from build123d import *

# Parameters (mm, degrees)
BOX015_W                  = 10
BOX015_H                  = 10
BOX015_DEPTH              = 19
BOX014_W                  = 10
BOX014_H                  = 10
BOX014_DEPTH              = 19
CHAMFER023006003002_SIZE2 = 9
CHAMFER023006003002_SIZE  = 10
TUBE_R                    = 4
TUBE_R_2                  = 2
TUBE_DEPTH                = 10


with BuildPart() as cube015:
    # Box015 → Box015 (new body)
    with BuildSketch(Plane(origin=(-8.5, 12, 8.5), x_dir=(1, 0, 0), z_dir=(0, 0, 1))):
        with Locations((5, 5)):
            Rectangle(BOX015_W, BOX015_H)
    extrude(amount=BOX015_DEPTH)


with BuildPart() as chamfer023006003002:
    # Box014 → Box014 (new body)
    with BuildSketch(Plane(origin=(-10.5, 0, 0), x_dir=(1, 0, 0), z_dir=(0, 0, 1))):
        with Locations((5, 5)):
            Rectangle(BOX014_W, BOX014_H)
    extrude(amount=BOX014_DEPTH)

    # Chamfer023006003002
    chamfer023006003002_edges = [chamfer023006003002.edges().sort_by_distance(p)[0] for p in [
        (-5.5, 10, 19),
    ]]
    chamfer023006003002_side = chamfer023006003002.faces().sort_by_distance((-5.5, 10, 9.5))[0]
    chamfer(chamfer023006003002_edges, length=CHAMFER023006003002_SIZE, length2=CHAMFER023006003002_SIZE2, reference=chamfer023006003002_side)


with BuildPart() as chamfer023006003002_1:
    # Chamfer023006003002 placement: moved
    add(chamfer023006003002.part.moved(Location((2, 2, 3.5))))


with BuildPart() as cut003001018:
    # Tube → Tube (new body)
    with BuildSketch(Plane(origin=(-3.5, 11, 12), x_dir=(1, 0, 0), z_dir=(0, 0, 1))):
        Circle(TUBE_R)
        Circle(TUBE_R_2, mode=Mode.SUBTRACT)
    extrude(amount=TUBE_DEPTH)

    # Cut003001017: cut Chamfer023006003002
    add(chamfer023006003002_1.part, mode=Mode.SUBTRACT)

    # Cut003001018: cut Cube015
    add(cube015.part, mode=Mode.SUBTRACT)


with BuildPart() as cut003001018_1:
    # Cut003001018 placement: moved
    add(cut003001018.part.moved(Location((0, 0, 0.5))))


solid = cut003001018_1.part
For this review, take the finished solid that the model builds, in its own axes (mm). Give positions to 0.01 mm unless a question says otherwise; leave off trailing zeros. Loops run counter-clockwise (first coordinate to the right, second up) from the corner with the lowest first, then second, coordinate; pieces in that order, holes last.
Item 1: Take a section at D-D, the plane x = -3.5. State the section outline as (y, z) points.
Item 2: Take a section at C-C, the plane z = 19. State the section outline as (x, y) points.
Item 3: For line 1 along X through (y, z) = (11, 20.75); line 2 along Y through (x, z) = (-3.5, 19.25); line 3 along X through (y, z) = (10.55, 21.75), list the stretches that pass through material, from the lowest coordinate up.
Item 4: Insertion check: pin 1 (1.5 mm diameter, centred on x = -2.5, y = 8.5, fed in from -Z); pin 2 (2 mm diameter, centred on x = -6.5, y = 8.5, fed in from -Z); pin 3 (4 mm diameter, centred on x = -0.5, z = 19, fed in from -Y). Each pin has a flat end and moves straight along its axis. Give the tip position at first contact, or say it passes through.
Item 5: Draft analysis for pull direction Y (two halves, no side actions). For faces 1 (the flat face through (-6, 12, 18)), 2 (the cylindrical face through (-3.56, 9, 18.74)), 3 (the flat face through (-4.4, 9, 22.5)), 4 (the flat face through (-4.445, 8.909, 16.434)), state which applies: +Y half, -Y half, draft (parallel to the pull), parting line (faces both ways), or undercut.
Item 6: Take a section at A-A, the plane y = 11. State the section outline as (x, z) points, and give its area (3 significant figures).
Item 7: Take a section at B-B, the plane z = 14.5. State the section outline as (x, y) points.
Calculated:
1. outline: (7, 18.56) - (9, 16.33) - (9, 22.5) - (7, 22.5) - close
2. outline: (-7.37, 12) arc R4 ccw (long way) to (0.37, 12) - (-1.77, 12) arc R2 cw (long way) to (-5.23, 12) - close
3. line 1: x = -7.5 to -5.5, -1.5 to 0.5
3. line 2: y = 7 to 9
3. line 3: x = -7.47 to -5.45, -1.55 to 0.47
4. pin 1: stops at z = 16.06
4. pin 2: stops at z = 15.78
4. pin 3: stops at y = 7.13
5. face 1: +Y half
5. face 2: undercut
5. face 3: draft
5. face 4: -Y half
6. outline: (-7.5, 14.11) - (-5.5, 14.11) - (-5.5, 22.5) - (-7.5, 22.5) - close; (-1.5, 14.11) - (0.5, 14.11) - (0.5, 22.5) - (-1.5, 22.5) - close
6. area: 33.6 mm2
7. outline: (-7.48, 10.65) - (-5.47, 10.65) arc R2 cw to (-5.23, 12) - (-7.37, 12) arc R4 ccw to start; (-1.77, 12) arc R2 cw to (-1.53, 10.65) - (0.48, 10.65) arc R4 ccw to (0.37, 12) - close
